Geometry: see drawing. Coordinates: mm, zero at the bounding-box minimum. Give positions to 0.01 mm unless a question says otherwise; leave off trailing zeros. Write each loop counter-clockwise with the first axis right and the second up, starting at its lowest first coordinate (ties: lowest second). Pieces come first, ordered by that corner, then holes. Notation, with made-up numbers: (56, 46.25) - (114, 46.25) arc R30 cw to (114, 74.25) - close; hole circle Ø7 at (-34.5, 12). An arc over 180 degrees is marked (long way). Use a Markdown table: item, result. Add a question column.
1. Section query A-A, the plane x = 192. Return loops of the section in (y, z) (1 decimal).
2. Section query D-D, the plane z = 90. Return loops of the section in (x, y), plus the area to 3 significant figures.
3. Section query B-B, the plane z = 339.5. Return loops of the section in (x, y), plus the area to 3 significant figures.
4. Section query C-C, the plane y = 4.75. Return loops of the section in (x, z) (1 decimal), plus the area to 3 significant figures.
5. Material intervals for probe 1 along Z at (x, y) = (188, 5); probe 2 along Z at (x, y) = (286.5, 18.5) (1 decimal); probe 3 along X at (y, z) = (12.5, 1201.5) (1 decimal), sorted ascending.
6. Pin query (flat end, axial travel): pin 1 (6 mm diameter, centred on y = 8.5, z = 898.5, fed in from -X); pin 2 (10 mm diameter, centred on y = 10.5, z = 835.5, fed in from +X); pin 3 (3 mm diameter, centred on x = 294, y = 6, fed in from -Z). Return the tip coordinate at first contact, or that it passes through.
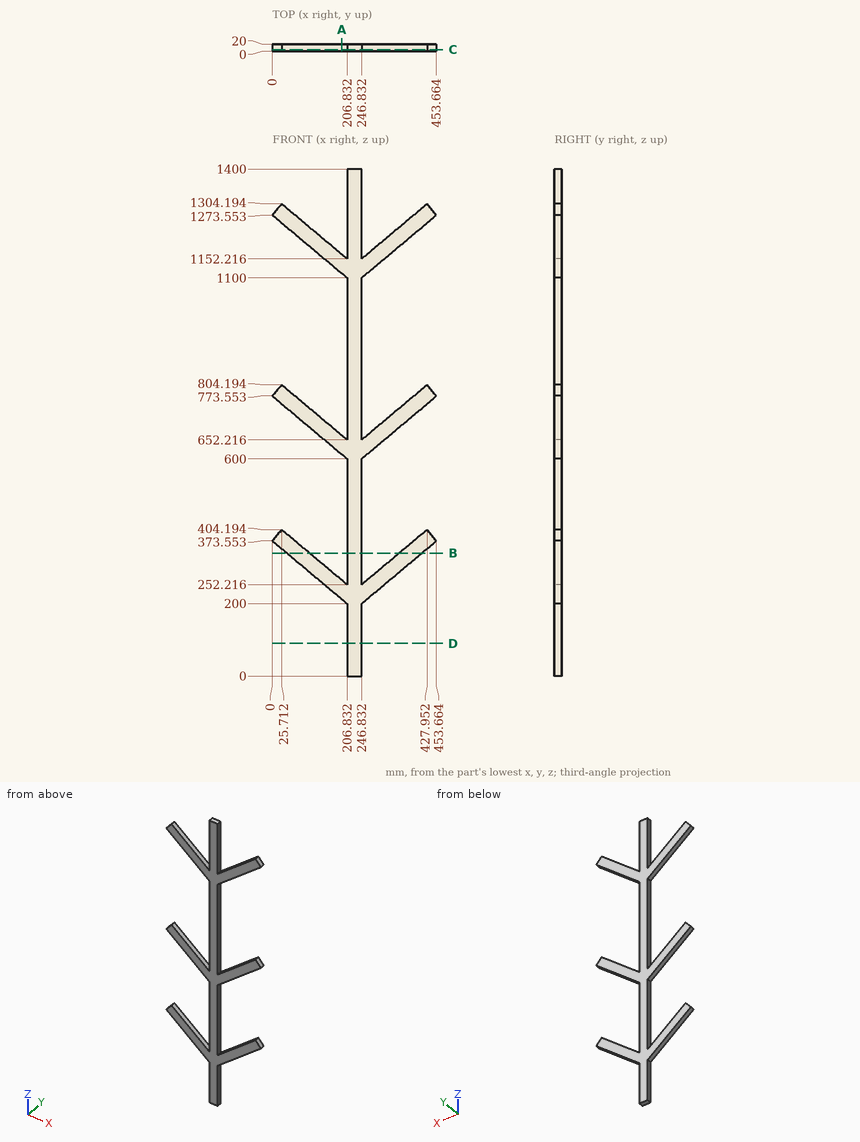
Result sheet:
| question | item | result |
|---|---|---|
| 1 | outline | (0, 212.4) - (20, 212.4) - (20, 264.7) - (0, 264.7) - close; (0, 612.4) - (20, 612.4) - (20, 664.7) - (0, 664.7) - close; (0, 1112.4) - (20, 1112.4) - (20, 1164.7) - (0, 1164.7) - close |
| 2 | outline | (206.83, 0) - (246.83, 0) - (246.83, 20) - (206.83, 20) - close |
| 2 | area | 800 mm² |
| 3 | outline | (40.58, 0) - (102.81, 0) - (102.81, 20) - (40.58, 20) - close; (206.83, 0) - (246.83, 0) - (246.83, 20) - (206.83, 20) - close; (350.85, 0) - (413.08, 0) - (413.08, 20) - (350.85, 20) - close |
| 3 | area | 3,290 mm² |
| 4 | outline | (0, 373.6) - (206.8, 200) - (206.8, 0) - (246.8, 0) - (246.8, 200) - (453.7, 373.6) - (428, 404.2) - (246.8, 252.2) - (246.8, 600) - (453.7, 773.6) - (428, 804.2) - (246.8, 652.2) - (246.8, 1100) - (453.7, 1273.6) - (428, 1304.2) - (246.8, 1152.2) - (246.8, 1400) - (206.8, 1400) - (206.8, 1152.2) - (25.7, 1304.2) - (0, 1273.6) - (206.8, 1100) - (206.8, 652.2) - (25.7, 804.2) - (0, 773.6) - (206.8, 600) - (206.8, 252.2) - (25.7, 404.2) - close |
| 4 | area | 117,000 mm² |
| 5 | probe 1 | z = 215.8 to 268.02, 615.8 to 668.02, 1115.8 to 1168.02 |
| 5 | probe 2 | z = 233.3 to 285.5, 633.3 to 685.5, 1133.3 to 1185.5 |
| 5 | probe 3 | x = 85.9 to 148.1, 206.8 to 246.8, 305.6 to 367.8 |
| 6 | pin 1 | stops at x = 206.83 |
| 6 | pin 2 | stops at x = 246.83 |
| 6 | pin 3 | stops at z = 238.32 |
